```python
from build123d import *

# Parameters (mm, degrees)
F0_R     = 19.05
F1_DEPTH = 5.08
F3_DEPTH = 12.7
F4_R     = 5.08
F5_R     = 19.05
F6_DEPTH = 5.08


with BuildPart() as f1:
    # F0 (on Front) → F1 (new body)
    with BuildSketch(Plane.XZ):
        Circle(F0_R)
    extrude(amount=F1_DEPTH)

    # F2 (on Right) → F3 (join, symmetric)
    with BuildSketch(Plane.YZ):
        with BuildLine():
            Line((-5.08, -12.7), (-5.08, 12.7))
            Line((-5.08, 12.7), (-43.18, 12.7))
            ThreePointArc((-43.18, 12.7), (-47.670128, 10.840128), (-49.53, 6.35))
            Line((-49.53, 6.35), (-49.53, -12.7))
            Line((-49.53, -12.7), (-49.53, -31.75))
            Line((-49.53, -31.75), (-24.13, -31.75))
            Line((-24.13, -31.75), (-24.13, -19.05))
            ThreePointArc((-24.13, -19.05), (-22.270128, -14.559872), (-17.78, -12.7))
            Line((-17.78, -12.7), (-5.08, -12.7))
        make_face()
    extrude(amount=F3_DEPTH, both=True)

    # F4
    f4_edges = [f1.edges().sort_by_distance(p)[0] for p in [
        (-12.7, -24.13, 12.7),
        (12.7, -24.13, 12.7),
        (12.7, -11.43, -12.7),
        (-12.7, -24.13, -25.4),
    ]]
    fillet(f4_edges, radius=F4_R)

    # F5 (on face) → F6 (join)
    with BuildSketch(Plane(origin=(0, 0, -31.75), x_dir=(1, 0, 0), z_dir=(0, 0, -1))):
        with Locations((0, 38.1)):
            Circle(F5_R)
    extrude(amount=F6_DEPTH)


solid = f1.part
```
CAD build for the part. Positions are in the model's coordinates, mm. A direction names the side the tool comes from. Round coordinates to 2 decimals unless told otherwise and drop trailing zeros. Loops run counter-clockwise (first coordinate to the right, second up) from the corner with the lowest first, then second, coordinate; pieces in that order, holes last. Notation, with made-up numbers: (50.5, 55.25) - (73.5, 55.25) arc R30 cw to (73.5, 86.25) - close; hole circle Ø3 at (22.5, 71). An arc over 180 degrees is marked (long way). Return JSON: item names as keys, results as strings. Group by question number.
Q1. Band-saw the part on A-A on x = 0. Give the cut face in (y, z).
Q2. Band-saw the part on D-D on x = 15.5. Give the cut face in (y, z).
Q3. Band-saw the part on B-B on y = -38.1. Give the cut face in (x, z), plus the area to 3 significant figures.
Q4. Band-saw the part on C-C on z = 0. Give the cut face in (x, y), plus the area to 3 significant figures.
Q5. Tool access for faces 5 (the face through (0, -24.13, -25)), 6 (the face through (12.7, -29, -7)), 7 (the face through (0, -49.53, -12)): list every direction of +Z, -Z, +X, -X, +Y, -Y with a clear straight run to the whole face (end or side of a thin tool).
Q6. Two-plate mould, pull along Z, no slides. Class faces 1 (the face through (-15.12, -2.5, -11.59)), 2 (the face through (-4.13, -19.503, -34.254)), 3 (the face through (-11.251, -25.658, -25.311)), 4 (the face through (11.172, -25.579, -25.311)): +Z half, -Z half, draft (parallel to the pull), parting line (faces both ways), or undercut.
Q7. Flat gauge pins, fed straight in: pin 1 Ø4.5 at (x, z) = (-1, -6.5) entering from -Y; pin 2 Ø1.5 at (y, z) = (-35, -7) entering from -X; pin 3 Ø4 at (y, z) = (-38.5, 0) entering from +X. Where does each tip first touch, or does it go through?
Q8. Drill centre lines: line 1 along Z through (x, y) = (-4, -16.5); line 2 along Y through (x, z) = (-4.5, -23); line 3 along Z through (x, y) = (-7.5, -25). Where is each one in solid material? Low to high. Write a range as [from, to].
Solutions:
{
 "1": {"outline": "(-57.15, -36.83) - (-19.05, -36.83) - (-19.05, -31.75) - (-24.13, -31.75) - (-24.13, -19.05) arc R6.35 cw to (-17.78, -12.7) - (-5.08, -12.7) - (-5.08, -19.05) - (0, -19.05) - (0, 19.05) - (-5.08, 19.05) - (-5.08, 12.7) - (-43.18, 12.7) arc R6.35 ccw to (-49.53, 6.35) - (-49.53, -31.75) - (-57.15, -31.75) - close"},
 "2": {"outline": "(-49.17, -36.83) - (-27.03, -36.83) - (-27.03, -31.75) - (-49.17, -31.75) - close; (-5.08, -11.07) - (0, -11.07) - (0, 11.07) - (-5.08, 11.07) - close"},
 "3": {"outline": "(-19.05, -36.83) - (19.05, -36.83) - (19.05, -31.75) - (12.7, -31.75) - (12.7, 7.62) arc R5.08 ccw to (7.62, 12.7) - (-7.62, 12.7) arc R5.08 ccw to (-12.7, 7.62) - (-12.7, -31.75) - (-19.05, -31.75) - close", "area": "1,310 mm^2"},
 "4": {"outline": "(-19.05, -5.08) - (-12.7, -5.08) - (-12.7, -44.45) arc R5.08 ccw to (-7.62, -49.53) - (7.62, -49.53) arc R5.08 ccw to (12.7, -44.45) - (12.7, -5.08) - (19.05, -5.08) - (19.05, 0) - (-19.05, 0) - close", "area": "1,310 mm^2"},
 "5": {"face 5": "+X, -X, +Y", "face 6": "+Z, +X, -Y", "face 7": "+Z, +X, -X, -Y"},
 "6": {"face 1": "parting line", "face 2": "draft", "face 3": "undercut", "face 4": "undercut"},
 "7": {"pin 1": "stops at y = -49.53", "pin 2": "stops at x = -12.7", "pin 3": "stops at x = 12.7"},
 "8": {"line 1": "z = [-12.7, 12.7]", "line 2": "y = [-49.53, -24.13]", "line 3": "z = [-36.83, 12.7]"}
}
